Work out the finished part from the listing and answer in its coordinate system (mm). A direction names the side the tool comes from. Coordinates: 2 decimals unless noted, no trailing zeros. Order: outer loops, then holes, each group sorted by start corner. A loop starts at its lowest first (then second) coordinate and runs counter-clockwise, first axis right, second up.
1. Find the intervals of material crossed by probe 1 along Y at (x, z) = (-6.25, -33); probe 2 along Z at (x, y) = (11, 7); probe 3 along Y at (x, z) = (-11.1, 28), in increasing order.
2. The part is cut by section C-C, the plane x = 0. Give the vertices of the cut face in (y, z), then the cut area to 3 significant figures.
3. Flat-ended cylindrical pins translate along their axes: pin 1 Ø21 at (x, y) = (-29, 25) entering from -Z; pin 2 Ø12 at (x, z) = (-16, 6) entering from -Y; pin 3 Ø2.5 at (x, z) = (13, -3.5) entering from +Y. Find the tip coordinate at first contact, or state that the pin passes through.
4. A tool of negligible diameter and unlimited length cuts with its end or side. For faces 1 (the flat face through (-11, 60, -7)), 2 (the flat face through (-60, 82, 0)), 3 (the cylindrical face through (10.03, 7.83, 30.48)), 4 (the flat face through (19, 11, -8)), from which of +Z, -Z, +X, -X, +Y, -Y can it reach the whole face along a straight path? Write none if from no direction.
5. Determine the mould class of faces 5 (the flat face through (-6, 19, -20)), 6 (the flat face through (15.5, 36, 0)) for opening direction Z: +Z half, -Z half, draft (parallel to the pull), parting line (faces both ways), or undercut.
6. The part is cut by section B-B, the plane z = -24. Give the vertices of the cut face in (x, y), then the cut area to 3 significant figures.
7. The part is cut by section D-D, the plane y = -37. Give the vertices of the cut face in (x, z), then the cut area to 3 significant figures.
8. The part is cut by section A-A, the plane y = 79.5. Give the vertices of the cut face in (x, z), then the cut area to 3 significant figures.
```python
from build123d import *

# Parameters (mm, degrees)
TYKKELSE_LEDDFESTER_OG_BREDDE_H_YDE_SELV_DEPTH = 13
SKETCH28_R                                     = 15.5
SKETCH28_R_2                                   = 10.5
HULL_TIL_L_RBEN_KARBONFIBERR_R_DEPTH           = 10
SKRUEHULL_LEDDFESTER_DEPTH                     = 167.325734629
SKRUEHULL_LEDDFESTER_DEPTH_BACK                = 167.325734629
SKETCH29_R                                     = 3
SKETCH33_W                                     = 5
SKETCH33_H                                     = 20
BREDDE_OG_AVSTAND_STEMPELENDE_DEPTH            = 60
CUT_EXTRUDE4_DEPTH                             = 148.147035308
SIDEM_NSTER_DEPTH                              = 7.650765
SIDEM_NSTER_2_DEPTH                            = 7.650765
UTVIDET_START                                  = -40
SKETCH44_R                                     = 10.5
UTVIDET_L_RBENHULL_INN_I_SELVE_KROPPEN_DEPTH   = 40
M_NSTER_TOPP_DEPTH                             = 10
STEMPELENDE_AV_ST_RSTE_SYLINDER_DEPTH          = 145.150962536
STEMPELENDE_AV_ST_RSTE_SYLINDER_DEPTH_BACK     = 145.150962536
ROD_ENDE_JUSTERE_LENGDEN_ALTS_FESTE_T_R        = 3
SKETCH39_W                                     = 5
SKETCH39_H                                     = 15
SYLINDERFESTE_SELVE_DEN_LILLE_SYLINDERE_DEPTH  = 25
ST_TTER_ST_RSTE_SYLINDER_1_DEPTH               = 5
ST_TTER_ST_RSTE_SYLINDER_2_DEPTH               = 5
SYLINDERFESTE_LITEN_SYLINDER_DEPTH             = 134.515916654
SYLINDERFESTE_LITEN_SYLINDER_DEPTH_BACK        = 134.515916654
SKETCH48_R                                     = 2.5
BOSS_EXTRUDE11_DEPTH                           = 5
BOSS_EXTRUDE12_DEPTH                           = 5
SKETCH51_R                                     = 10
TIL_ASSEMBLY_SLETT_F_R_PRINTING_DEPTH          = 170


with BuildPart() as part:
    # Sketch27 → Tykkelse leddfester og bredde/høyde selve modellen (new, symmetric)
    with BuildSketch(Plane.XY):
        Polygon((66, 0), (-66, 0), (-66, 100), (-60, 100), (-60, 70), (60, 70), (60, 100), (66, 100), align=None)
    extrude(amount=TYKKELSE_LEDDFESTER_OG_BREDDE_H_YDE_SELV_DEPTH, both=True)

    # Sketch28 → Hull til lårben/karbonfiberrør (add)
    with BuildSketch(Plane.XZ):
        with Locations(Location((0, 0, 0), (0, 0, 57.004114526))):
            Circle(SKETCH28_R)
        with Locations(Location((0, 0, 0), (0, 0, 270))):
            Circle(SKETCH28_R_2, mode=Mode.SUBTRACT)
    extrude(amount=HULL_TIL_L_RBEN_KARBONFIBERR_R_DEPTH)

    # Sketch29 → Skruehull leddfester (cut, two sides: drawn at the far end of the back side and taken through both)
    with BuildSketch(Plane(origin=(66, 0, 0), x_dir=(0, 0, -1), z_dir=(1, 0, 0)).offset(-SKRUEHULL_LEDDFESTER_DEPTH_BACK)):
        with Locations((0, 86.5)):
            Circle(SKETCH29_R)
        with BuildLine():
            Line((-13, 86.5), (-13, 71.5))
            Line((-13, 71.5), (-14, 71.5))
            Line((-14, 71.5), (-14, 101))
            Line((-14, 101), (0, 101))
            Line((0, 101), (14, 101))
            Line((14, 101), (14, 71.5))
            Line((14, 71.5), (13, 71.5))
            Line((13, 71.5), (13, 86.5))
            ThreePointArc((13, 86.5), (0, 99.5), (-13, 86.5))
        make_face()
    extrude(amount=SKRUEHULL_LEDDFESTER_DEPTH + SKRUEHULL_LEDDFESTER_DEPTH_BACK, mode=Mode.SUBTRACT)

    # Sketch33 → Bredde og avstand stempelende (add)
    with BuildSketch(Plane(origin=(0, 0, -13), x_dir=(-1, 0, 0), z_dir=(0, 0, -1))):
        with Locations((-6, 10)):
            Rectangle(SKETCH33_W, SKETCH33_H)
        with Locations((6, 10)):
            Rectangle(SKETCH33_W, SKETCH33_H)
    extrude(amount=BREDDE_OG_AVSTAND_STEMPELENDE_DEPTH)

    # Fasong (mønster på selve kroppen) → Cut-Extrude4 (cut, through all)
    with BuildSketch(Plane.XY.offset(13)):
        Polygon((-66, 60), (-15.5, 0), (-66, 0), align=None)
        Polygon((15.5, 0), (66, 0), (66, 60), align=None)
        Polygon((-56, 60), (-15.5, 11.881188119), (-15.5, 60), align=None)
        Polygon((56, 60), (15.5, 60), (15.5, 11.881188119), align=None)
    extrude(amount=-CUT_EXTRUDE4_DEPTH, mode=Mode.SUBTRACT)

    # Sketch40 → Sidemønster (cut)
    with BuildSketch(Plane(origin=(-9.072801919, -7.636274948, 0), x_dir=(0, 0, 1), z_dir=(-0.765076505498557, -0.6439393921279521, 0))):
        Polygon((-8, 81.90459021), (8, 81.90459021), (8, 65.90459021), align=None)
        Polygon((-8, 74.833522398), (8, 58.833522398), (-8, 42.833522398), align=None)
        Polygon((8, 19.762454587), (-8, 35.762454587), (8, 51.762454587), align=None)
        Polygon((-8, 28.691386775), (8, 12.691386775), (-8, 12.691386775), align=None)
    extrude(amount=-SIDEM_NSTER_DEPTH, mode=Mode.SUBTRACT)

    # Sketch42 → Sidemønster 2 (cut)
    with BuildSketch(Plane(origin=(9.072801919, -7.636274948, 0), x_dir=(0, 0, -1), z_dir=(0.765076505498557, -0.6439393921279521, 0))):
        Polygon((8, 81.90459021), (-8, 81.90459021), (-8, 65.90459021), align=None)
        Polygon((8, 74.833522398), (-8, 58.833522398), (8, 42.833522398), align=None)
        Polygon((-8, 51.762454587), (8, 35.762454587), (-8, 19.762454587), align=None)
        Polygon((8, 28.691386775), (-8, 12.691386775), (8, 12.691386775), align=None)
    extrude(amount=-SIDEM_NSTER_2_DEPTH, mode=Mode.SUBTRACT)

    # Sketch44 → Utvidet lårbenhull inn i selve kroppen (cut)
    with BuildSketch(Plane.XZ.offset(UTVIDET_START)):
        with Locations(Location((0, 0, 0), (0, 0, 270))):
            Circle(SKETCH44_R)
    extrude(amount=UTVIDET_L_RBENHULL_INN_I_SELVE_KROPPEN_DEPTH, mode=Mode.SUBTRACT)

    # Sketch45 → Mønster topp (cut)
    with BuildSketch(Plane(origin=(0, 70, 0), x_dir=(1, 0, 0), z_dir=(0, 1, 0))):
        Polygon((-39.928932188, 10.5), (-31.928932188, 2.5), (-23.928932188, 10.5), align=None)
        Polygon((-16.857864376, 10.5), (-8.857864376, 2.5), (-8.857864376, 10.5), align=None)
        Polygon((-55, 2.5), (-55, 10.5), (-47, 10.5), align=None)
        Polygon((-43.464466094, 10.5), (-51.464466094, 2.5), (-35.464466094, 2.5), align=None)
        Polygon((-20.393398282, 10.5), (-28.393398282, 2.5), (-12.393398282, 2.5), align=None)
        Polygon((-8.857864376, -2.5), (-8.857864376, -10.5), (-16.857864376, -10.5), align=None)
        Polygon((-20.393398282, -10.5), (-12.393398282, -2.5), (-28.393398282, -2.5), align=None)
        Polygon((-23.928932188, -10.5), (-31.928932188, -2.5), (-39.928932188, -10.5), align=None)
        Polygon((-43.464466094, -10.5), (-35.464466094, -2.5), (-51.464466094, -2.5), align=None)
        Polygon((-55, -10.5), (-47, -10.5), (-55, -2.5), align=None)
        Polygon((8.857864376, 2.5), (8.857864376, 10.5), (16.857864376, 10.5), align=None)
        Polygon((16.857864376, -10.5), (8.857864376, -2.5), (8.857864376, -10.5), align=None)
        Polygon((20.393398282, -10.5), (28.393398282, -2.5), (12.393398282, -2.5), align=None)
        Polygon((20.393398282, 10.5), (12.393398282, 2.5), (28.393398282, 2.5), align=None)
        Polygon((23.928932188, 10.5), (31.928932188, 2.5), (39.928932188, 10.5), align=None)
        Polygon((23.928932188, -10.5), (39.928932188, -10.5), (31.928932188, -2.5), align=None)
        Polygon((43.464466094, -10.5), (51.464466094, -2.5), (35.464466094, -2.5), align=None)
        Polygon((55, -2.5), (55, -10.5), (47, -10.5), align=None)
        Polygon((43.464466094, 10.5), (35.464466094, 2.5), (51.464466094, 2.5), align=None)
        Polygon((55, 10.5), (47, 10.5), (55, 2.5), align=None)
    extrude(amount=-M_NSTER_TOPP_DEPTH, mode=Mode.SUBTRACT)

    # Rod-ende, justere lengden (altså feste til største sylinder) → Stempelende av st_rste sylinder (cut, two sides: drawn at the far end of the back side and taken through both)
    with BuildSketch(Plane(origin=(8.5, 0, 0), x_dir=(0, 0, -1), z_dir=(1, 0, 0)).offset(-STEMPELENDE_AV_ST_RSTE_SYLINDER_DEPTH_BACK)):
        with Locations((33, 10)):
            Circle(ROD_ENDE_JUSTERE_LENGDEN_ALTS_FESTE_T_R)
        with BuildLine():
            Line((43, -1), (74, -1))
            Line((74, -1), (74, 21))
            Line((74, 21), (43, 21))
            Line((43, 21), (13, 21))
            Line((13, 21), (13, 19))
            Line((13, 19), (33, 19))
            ThreePointArc((33, 19), (42, 10), (33, 1))
            Line((33, 1), (13, 1))
            Line((13, 1), (13, -1))
            Line((13, -1), (43, -1))
        make_face()
    extrude(amount=STEMPELENDE_AV_ST_RSTE_SYLINDER_DEPTH + STEMPELENDE_AV_ST_RSTE_SYLINDER_DEPTH_BACK, mode=Mode.SUBTRACT)

    # Sketch39 → Sylinderfeste_ selve den lille sylindere (add)
    with BuildSketch(Plane.XY.offset(13)):
        with Locations((-10, 7.5)):
            Rectangle(SKETCH39_W, SKETCH39_H)
        with Locations((10, 7.5)):
            Rectangle(SKETCH39_W, SKETCH39_H)
    extrude(amount=SYLINDERFESTE_SELVE_DEN_LILLE_SYLINDERE_DEPTH)

    # Sketch46 → Støtter største sylinder 1 (add)
    with BuildSketch(Plane(origin=(8.5, 0, 0), x_dir=(0, 0, -1), z_dir=(1, 0, 0))):
        Polygon((13, 44), (13, 35.996094703), (26.596875763, 19), (33, 19), align=None)
    extrude(amount=-ST_TTER_ST_RSTE_SYLINDER_1_DEPTH)

    # Sketch47 → Støtter største sylinder 2 (add)
    with BuildSketch(Plane.ZY.offset(8.5)):
        Polygon((-33, 19), (-13, 44), (-13, 35.996094703), (-26.596875763, 19), align=None)
    extrude(amount=-ST_TTER_ST_RSTE_SYLINDER_2_DEPTH)

    # Sketch48 → Sylinderfeste, liten sylinder (cut, two sides: drawn at the far end of the back side and taken through both)
    with BuildSketch(Plane.ZY.offset(12.5).offset(-SYLINDERFESTE_LITEN_SYLINDER_DEPTH_BACK)):
        with Locations(Location((28, 7.5, 0), (0, 0, 270))):
            Circle(SKETCH48_R)
        with BuildLine():
            Line((28, 0), (13.179811187, 0))
            Line((13.179811187, 0), (13.179811187, -1))
            Line((13.179811187, -1), (39, -1))
            Line((39, -1), (39, 16))
            Line((39, 16), (13, 16))
            Line((13, 16), (13, 15))
            Line((13, 15), (28, 15))
            ThreePointArc((28, 15), (35.5, 7.5), (28, 0))
        make_face()
    extrude(amount=SYLINDERFESTE_LITEN_SYLINDER_DEPTH + SYLINDERFESTE_LITEN_SYLINDER_DEPTH_BACK, mode=Mode.SUBTRACT)

    # Sketch49 → Boss-Extrude11 (add)
    with BuildSketch(Plane.ZY.offset(12.5)):
        Polygon((28, 15), (13, 40), (13, 30.281746842), (22.169048105, 15), align=None)
    extrude(amount=-BOSS_EXTRUDE11_DEPTH)

    # Sketch50 → Boss-Extrude12 (add)
    with BuildSketch(Plane(origin=(12.5, 0, 0), x_dir=(0, 0, -1), z_dir=(1, 0, 0))):
        Polygon((-28, 15), (-22.169048105, 15), (-13, 30.281746842), (-13, 40), align=None)
    extrude(amount=-BOSS_EXTRUDE12_DEPTH)

    # Sketch51 → TIL ASSEMBLY - SLETT FØR PRINTING (add)
    with BuildSketch(Plane.XZ.offset(-40)):
        with Locations(Location((0, 0, 0), (0, 0, 270))):
            Circle(SKETCH51_R)
    extrude(amount=TIL_ASSEMBLY_SLETT_F_R_PRINTING_DEPTH)


solid = part.part
```
Geometry says:
1. probe 1: y = 1 to 7, 13 to 19
1. probe 2: z = -13 to 25.55, 30.45 to 35.48
1. probe 3: y = 0 to 5, 10 to 15
2. outline: (-130, -10) - (40, -10) - (40, -10.5) - (-10, -10.5) - (-10, -15.5) - (-1, -15.5) - (-1, -13) - (70, -13) - (70, 13) - (0, 13) - (0, 13.18) - (-1, 13.18) - (-1, 15.5) - (-10, 15.5) - (-10, 10.5) - (40, 10.5) - (40, 10) - (-130, 10) - close
2. area: 4,480 mm2
3. pin 1: stops at z = -13
3. pin 2: stops at y = -10
3. pin 3: stops at y = 70
4. face 1: +Y
4. face 2: +Z, -Z, +Y
4. face 3: +X, -X
4. face 4: none
5. face 5: undercut
5. face 6: draft
6. outline: (-8.5, 1) - (-3.5, 1) - (-3.5, 19) - (-8.5, 19) - close; (-8.5, 22.25) - (-3.5, 22.25) - (-3.5, 30.25) - (-8.5, 30.25) - close; (3.5, 1) - (8.5, 1) - (8.5, 19) - (3.5, 19) - close; (3.5, 22.25) - (8.5, 22.25) - (8.5, 30.25) - (3.5, 30.25) - close
6. area: 260 mm2
7. outline: circle Ø20 at (0, 0)
7. area: 314 mm2
8. outline: (-66, -13) - (-60, -13) - (-60, 13) - (-66, 13) - close; (60, -13) - (66, -13) - (66, 13) - (60, 13) - close
8. area: 312 mm2
